```python
from build123d import *

# Parameters (mm, degrees)
SKETCH1_R           = 6.2
BOSS_EXTRUDE1_DEPTH = 19.5
SKETCH2_R           = 2
BOSS_EXTRUDE2_DEPTH = 2.8
SKETCH3_W           = 0.9633
SKETCH3_H           = 5.7798
BOSS_EXTRUDE3_DEPTH = 2.8


with BuildPart() as part:
    # Sketch1 → Boss-Extrude1 (new body)
    with BuildSketch(Plane(origin=(0, 0, 0), x_dir=(1, 0, 0), z_dir=(0, 1, 0))):
        with Locations(Location((0, 0, 0), (0, 0, 270))):
            Circle(SKETCH1_R)
    extrude(amount=BOSS_EXTRUDE1_DEPTH)

    # Sketch2 → Boss-Extrude2 (add)
    with BuildSketch(Plane(origin=(0, 19.5, 0), x_dir=(1, 0, 0), z_dir=(0, 1, 0))):
        with Locations(Location((0, 0, 0), (0, 0, 270))):
            Circle(SKETCH2_R)
    extrude(amount=BOSS_EXTRUDE2_DEPTH)

    # Sketch3 → Boss-Extrude3 (add)
    with BuildSketch(Plane.XZ):
        with Locations((4.78885, 0)):
            Rectangle(SKETCH3_W, SKETCH3_H)
        with Locations((-4.78885, 0)):
            Rectangle(SKETCH3_W, SKETCH3_H)
    extrude(amount=BOSS_EXTRUDE3_DEPTH)


solid = part.part
```
Model file for the job. Use its own axes, mm. A direction names the side the tool comes from. Round coordinates to 2 decimals unless told otherwise and drop trailing zeros. Write each loop counter-clockwise with the first axis right and the second up, starting at its lowest first coordinate (ties: lowest second). Pieces come first, ordered by that corner, then holes. Notation, with made-up numbers: (-14, 66.25) - (12, 66.25) arc R17 ccw to (12, 73.25) - close; hole circle Ø4 at (23.5, -27). An arc over 180 degrees is marked (long way). Use CSV: the item, a comma, the result in double quotes. Start each with the question number.
Item 1: Drill centre lines: L1, parallel to X at y = 3.25, z = 0.25; L2, parallel to Y at x = 0, z = -0.25; L3, parallel to Y at x = -0.25, z = 3.75. Where is each one in solid material? Low to high. Write a range as [from, to].
Item 2: Band-saw the part on B-B (z = 0). Write the cut outline in (x, y), and give its area (3 significant figures).
Item 3: Band-saw the part on A-A (y = -1). Write the cut outline in (x, z).
Item 4: Two-plate mould, pull along X, no slides. Class faces 5 (the face through (-4.307, -1, 0)), 6 (the face through (1.9, 9.6, 5.9)), 7 (the face through (-5, -2.8, 0)): released by +X, released by -X, zero draft, split by the parting line, or undercut.
Item 5: Tool access for faces 1 (the face through (4.307, -1, 0)), 2 (the face through (5.27, -1, 0)), 3 (the face through (-5, -1, -2.89)), 4 (the face through (-5, -1, 2.89)): list every direction of +Z, -Z, +X, -X, +Y, -Y with a clear straight run to the whole face (end or side of a thin tool).
Item 6: Pin check, flat tips, straight feed: P1, Ø1.5, axis at x = -1.5, y = 10.5, coming from the +Z side; P2, Ø1.5, axis at x = -1.5, y = 19.5, coming from the -Z side; P3, Ø1.5, axis at x = -0.5, z = -3, coming from the +Y side; P4, Ø2, axis at x = -4, z = -3.5, coming from the -Y side. Stop position of each tip, or through.
Item 7: Band-saw the part on C-C (x = 0). Write the cut outline in (y, z), and give its area (3 significant figures).
Item 8: Band-saw the part on D-D (y = 18). Write the cut outline in (x, z), and give its area (3 significant figures).
Checked values:
1,L1,"x = [-6.19, 6.19]"
1,L2,"y = [0, 22.3]"
1,L3,"y = [0, 19.5]"
2,outline,"(-6.2, 0) - (-5.27, 0) - (-5.27, -2.8) - (-4.31, -2.8) - (-4.31, 0) - (4.31, 0) - (4.31, -2.8) - (5.27, -2.8) - (5.27, 0) - (6.2, 0) - (6.2, 19.5) - (2, 19.5) - (2, 22.3) - (-2, 22.3) - (-2, 19.5) - (-6.2, 19.5) - close"
2,area,"258 mm²"
3,outline,"(-5.27, -2.89) - (-4.31, -2.89) - (-4.31, 2.89) - (-5.27, 2.89) - close; (4.31, -2.89) - (5.27, -2.89) - (5.27, 2.89) - (4.31, 2.89) - close"
4,face 5,"undercut"
4,face 6,"split by the parting line"
4,face 7,"zero draft"
5,face 1,"+Z, -Z, -Y"
5,face 2,"+Z, -Z, +X, -Y"
5,face 3,"-Z, +X, -X, -Y"
5,face 4,"+Z, +X, -X, -Y"
6,P1,"stops at z = 6.15"
6,P2,"stops at z = -6.15"
6,P3,"stops at y = 19.5"
6,P4,"stops at y = -2.8"
7,outline,"(0, -6.2) - (19.5, -6.2) - (19.5, -2) - (22.3, -2) - (22.3, 2) - (19.5, 2) - (19.5, 6.2) - (0, 6.2) - close"
7,area,"253 mm²"
8,outline,"circle Ø12.4 at (0, 0)"
8,area,"121 mm²"
